Read the model definition and answer for the solid it produces. Units are mm, in the model's axes. Give positions to 0.01 mm unless a question says otherwise; leave off trailing zeros. Order: outer loops, then holes, each group sorted by start corner. A loop starts at its lowest first (then second) coordinate and runs counter-clockwise, first axis right, second up. Notation, with made-up numbers: (81, 3) - (95, 3) arc R20 cw to (95, 33) - close; hole circle Ø8 at (72.5, 69.25). An arc over 180 degrees is marked (long way). Write each question's results on one line, items separated by ' | '.
Autodesk Inventor part; units mm, degrees
ref_plane "YZ Plane" through (0, 0, 0) normal (1, 0, 0) x (0, 1, 0)
ref_plane "XZ Plane" through (0, 0, 0) normal (0, 1, 0) x (-1, 0, 0)
ref_plane "XY Plane" through (0, 0, 0) normal (0, 0, 1) x (1, 0, 0)
sketch "Skizze1" plane through (0, 0, 0) normal (0, 1, 0) x (-1, 0, 0)
  line L0 (-10, 30) -> (10, 30)
  line L1 (10, 30) -> (10, -30)
  line L2 (10, -30) -> (-10, -30)
  line L3 (-10, -30) -> (-10, 30)
  line L4 (-10, 30) -> (10, -30) construction
  line L5 (10, 30) -> (-10, -30) construction
  circle A0 centre (0, 20) radius 1
  point P0 (0, 0)
  point P1 (0, 0)
  dimension "d0" = 60
  dimension "d1" = 20
  dimension "d2" = 2
  dimension "d3" = 10
extrude "Extrusion1" add sketch "Skizze1" along normal blind 2
properties part number "Grundplatte"
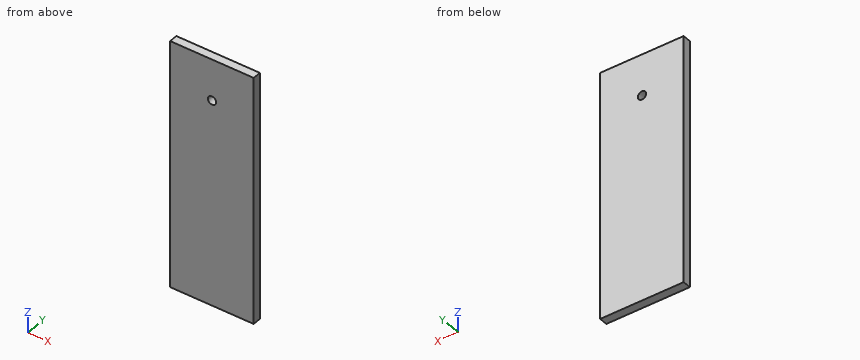
(1) Section B-B (z = 20) is taken. Give the vertices of the cut face in (x, y), plus the area to 3 significant figures.
Conclusion:
outline: (-10, 0) - (-1, 0) - (-1, 2) - (-10, 2) - close; (1, 0) - (10, 0) - (10, 2) - (1, 2) - close | area: 36.0 mm^2
(2) Section A-A (x = 0) is taken. Give the vertices of the cut face in (y, z), plus the area to 3 significant figures.
Conclusion:
outline: (0, -30) - (2, -30) - (2, 19) - (0, 19) - close; (0, 21) - (2, 21) - (2, 30) - (0, 30) - close | area: 116 mm^2
(3) Consider probe 1 along Z at (x, y) = (0, 0.65); probe 2 along Z at (x, y) = (-0.5, 0.75). Determine where each line is inside the solid, lowest interval first. Write a range as [from, to].
Conclusion:
probe 1: [-30, 19], [21, 30] | probe 2: [-30, 19.13], [20.87, 30]
